The listing builds one solid part. Answer for the finished solid, in the listing's coordinates (mm). Face numbers are marked on the shaded views. Give positions to 0.01 mm unless a question says otherwise; leave off trailing zeros. Order: outer loops, then holes, each group sorted by start corner. A loop starts at its lowest first (then second) coordinate and runs counter-clockwise, first axis right, second up. Notation, with made-up numbers: (-33.5, -30) - (-25.5, -30) arc R22 cw to (-25.5, -20) - close; hole circle Ø9 at (-35.5, 43). An arc over 180 degrees is marked (long way). Use a Markdown table: item, result. Add a question column.
1) Find section A-A, the plane x = 166.5. Determine the outline of the cut face in (y, z) (3 decimals).
2) The mould has two halves that part along X. Classify the marked faces 1, 2 and 3: released by +X, released by -X, zero draft, split by the parting line, or undercut.
3) A flat-ended cylindrical pin translates along its axis: pin 1 (1.5 mm diameter, centred on y = 19, z = 16, fed in from -X). Find the tip coordinate at first contact, or state that the pin passes through.
4) Straight lines are drawn through the part: line 1 (Y direction, x = 91.5, z = 12.25); line 2 (Y direction, x = 106.5, z = 16.5) (3 decimals); line 3 (Z direction, x = 238, y = 61) (3 decimals). For each, find the intervals that lie inside material, in ascending order.
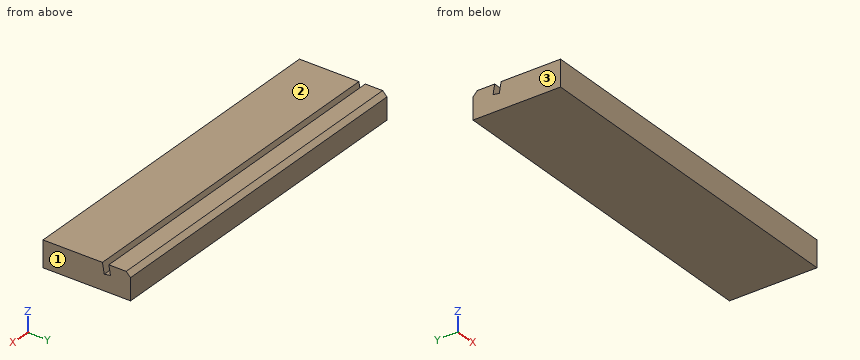
from build123d import *

# Parameters (mm, degrees)
F0_W     = 63.5
F0_H     = 19.05
F1_DEPTH = 254
F2_SIZE  = 3.175
F4_DEPTH = 254.001


with BuildPart() as f1:
    # F0 (on Right) → F1 (new body)
    with BuildSketch(Plane.YZ):
        with Locations((31.75, 9.525)):
            Rectangle(F0_W, F0_H)
    extrude(amount=F1_DEPTH)

    # F2
    f2_edges = [f1.edges().sort_by_distance(p)[0] for p in [
        (127, 63.5, 19.05),
    ]]
    chamfer(f2_edges, length=F2_SIZE)

    # F3 (on face) → F4 (cut, through all)
    with BuildSketch(Plane.YZ.offset(254)):
        Polygon((45.888826, 29.599109), (41.386285, 28.80519), (44.45, 11.43), (48.952541, 12.223919), align=None)
    extrude(amount=-F4_DEPTH, mode=Mode.SUBTRACT)


with BuildPart() as f5_1:
    # F5: copy of F1
    add(f1.part.moved(Location((0, 0, 82.55))))


with BuildPart() as f6_1:
    # F6: copy of F1
    add(f1.part.moved(Location((0, 0, 165.1))))


with BuildPart() as f7_1:
    # F7: copy of F1
    add(f1.part.moved(Location((0, 0, 247.65))))


solid = f1.part
The answers:
| question | item | result |
|---|---|---|
| 1 | outline | (0, 0) - (63.5, 0) - (63.5, 15.875) - (60.325, 19.05) - (47.749, 19.05) - (48.953, 12.224) - (44.45, 11.43) - (43.106, 19.05) - (0, 19.05) - close |
| 2 | face 1 | released by +X |
| 2 | face 2 | zero draft |
| 2 | face 3 | released by -X |
| 3 | pin 1 | x = 0 |
| 4 | line 1 | 0 to 44.31, 48.95 to 63.5 |
| 4 | line 2 | 0 to 43.556, 48.199 to 62.875 |
| 4 | line 3 | 0 to 18.375 |
